Read the model definition and answer for the solid it produces. Units are mm, in the model's axes. Round coordinates to 2 decimals unless told otherwise and drop trailing zeros. Write each loop counter-clockwise with the first axis right and the second up, starting at its lowest first coordinate (ties: lowest second). Pieces come first, ordered by that corner, then holes. Notation, with made-up numbers: (88, 74.5) - (101, 74.5) arc R17 ccw to (101, 100.5) - close; hole circle Ø1 at (53, 57.25). An arc over 180 degrees is marked (long way). One line per item, written item: value. Start each with the question number.
(1) A cutting plane is placed at A-A, the plane x = -68.58. Determine the outline of the cut face in (y, z) (3 decimals).
(2) Flat-ended cylindrical pins translate along their axes: pin 1 Ø10 at (x, z) = (48.49, 48.49) entering from -Y; pin 2 Ø4 at (x, z) = (0, -68.58) entering from +Y. Find the tip coordinate at first contact, or state that the pin passes through.
(3) Find the intervals of material crossed by L1, parallel to Z at x = 3.5, y = 4; L2, parallel to X at y = 2.5, z = -68.58 (3 decimals); L3, parallel to X at y = 5.75, z = 46, in increasing order.
(4) A cutting plane is placed at B-B, the plane z = -68.58. Determine the outline of the cut face in (x, y) (3 decimals), plus the area to 3 significant figures.
(5) A cutting plane is placed at C-C, the plane y = 1.5. State how many separate pieces and enclosed holes the cut face has, plus the area to 3 significant figures.
(6) A cutting plane is placed at D-D, the plane z = -51. Determine the outline of the cut face in (x, y).
from build123d import *

# Parameters (mm, degrees)
SKETCH1_R           = 3.175
SKETCH1_R_2         = 2
BOSS_EXTRUDE1_DEPTH = 6.35


with BuildPart() as part:
    # Sketch1 → Boss-Extrude1 (new body)
    with BuildSketch(Plane(origin=(0, 0, 0), x_dir=(1, 0, 0), z_dir=(0, 1, 0))):
        with BuildLine():
            Line((-33.21480995, -68.58), (33.21480995, -68.58))
            ThreePointArc((33.21480995, -68.58), (64.565503631, -40.46894786), (76.2, 0))
            ThreePointArc((76.2, 0), (-40.46894786, 64.565503631), (-33.21480995, -68.58))
        make_face()
        with Locations(Location((-48.493383054, -48.493383054, 0), (0, 0, 270))):
            Circle(SKETCH1_R, mode=Mode.SUBTRACT)
        with Locations(Location((-5.0038, -33.563454663, 0), (0, 0, 270))):
            Circle(SKETCH1_R_2, mode=Mode.SUBTRACT)
        with Locations(Location((48.493383054, -48.493383054, 0), (0, 0, 270))):
            Circle(SKETCH1_R, mode=Mode.SUBTRACT)
        with Locations(Location((5.0038, -33.563454663, 0), (0, 0, 270))):
            Circle(SKETCH1_R_2, mode=Mode.SUBTRACT)
        with Locations(Location((-68.58, 0, 0), (0, 0, 270))):
            Circle(SKETCH1_R, mode=Mode.SUBTRACT)
        with Locations(Location((-5.0038, 15.941145337, 0), (0, 0, 270))):
            Circle(SKETCH1_R_2, mode=Mode.SUBTRACT)
        with Locations(Location((5.0038, 15.941145337, 0), (0, 0, 270))):
            Circle(SKETCH1_R_2, mode=Mode.SUBTRACT)
        with Locations(Location((68.58, 0, 0), (0, 0, 270))):
            Circle(SKETCH1_R, mode=Mode.SUBTRACT)
        with Locations(Location((0, 68.58, 0), (0, 0, 270))):
            Circle(SKETCH1_R, mode=Mode.SUBTRACT)
    extrude(amount=BOSS_EXTRUDE1_DEPTH)


solid = part.part
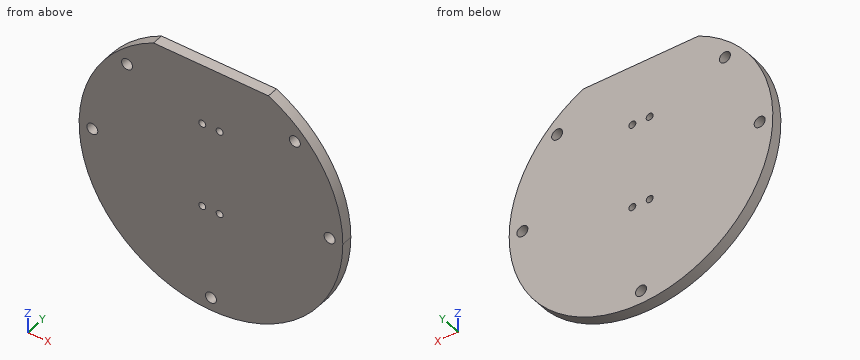
Here are the results:
1. outline: (0, -33.215) - (6.35, -33.215) - (6.35, -3.175) - (0, -3.175) - close; (0, 3.175) - (6.35, 3.175) - (6.35, 33.215) - (0, 33.215) - close
2. pin 1: y = 0
2. pin 2: through
3. L1: -76.12 to -17.26, -14.62 to 32.24, 34.88 to 68.58
3. L2: -33.215 to -3.175, 3.175 to 33.215
3. L3: -60.75 to -50.46, -46.53 to 46.53, 50.46 to 60.75
4. outline: (-33.215, 0) - (-3.175, 0) - (-3.175, 6.35) - (-33.215, 6.35) - close; (3.175, 0) - (33.215, 0) - (33.215, 6.35) - (3.175, 6.35) - close
4. area: 382 mm²
5. separate pieces: 1
5. enclosed holes: 9
5. area: 17,700 mm²
6. outline: (-56.62, 0) - (56.62, 0) - (56.62, 6.35) - (-56.62, 6.35) - close
